Study the drawing (mm; zero at the part's minimum x, y, z) and answer. A direction names the side the tool comes from. Round coordinates to 2 decimals unless told otherwise and drop trailing zeros. Loops run counter-clockwise (first coordinate to the right, second up) from the corner with the lowest first, then second, coordinate; pieces in that order, holes last. Notation, with made-up numbers: M 46.25,42 L 71.25,42 A14 cw 71.25,59 Z; hole C -22.5,-15.75 d9. An arc over 180 degrees is marked long. Write each question's results on one line, items separated by ' | '.
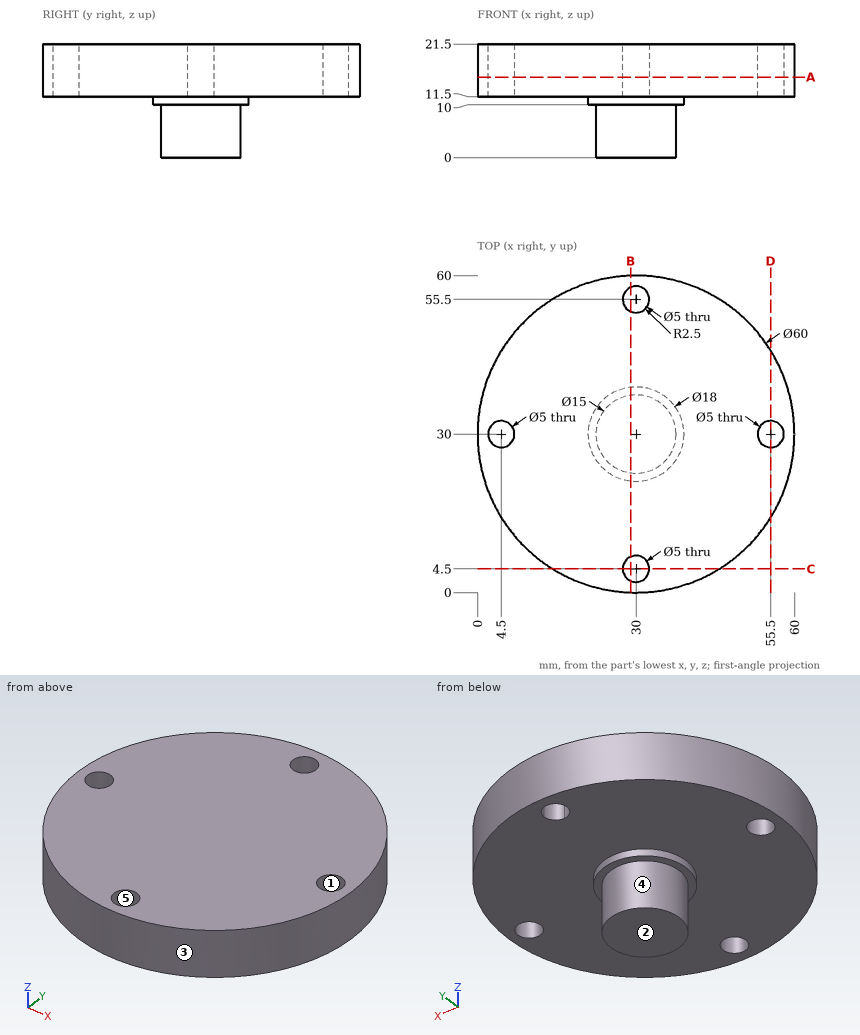
Item 1: For the marked faces 4 and 5, determine the directions among +Z, -Z, +X, -X, +Y, -Y from which every point of the face is accessible in a straight line to the end or side of a thin tool.
Outcome:
face 4: -Z | face 5: +Z, -Z
Item 2: The part is cut by section A-A (z = 15.25). Determine the outline of the cut face in (x, y).
Outcome:
outline: C 30,30 d60; hole C 4.5,30 d5; hole C 30,4.5 d5; hole C 30,55.5 d5; hole C 55.5,30 d5
Item 3: Straight lines are drawn through the part: line 1 (Y direction, x = 32, z = 12); line 2 (Z direction, x = 55, y = 27.5); line 3 (Y direction, x = 4.5, z = 16). For each, find the intervals that lie inside material, in ascending order.
Outcome:
line 1: y = 0.07 to 3, 6 to 54, 57 to 59.93 | line 2: z = 11.5 to 21.5 | line 3: y = 14.2 to 27.5, 32.5 to 45.8
Item 4: The part is cut by section C-C (y = 4.5). Determine the outline of the cut face in (x, z).
Outcome:
outline: M 14.2,11.5 L 27.5,11.5 L 27.5,21.5 L 14.2,21.5 Z; M 32.5,11.5 L 45.8,11.5 L 45.8,21.5 L 32.5,21.5 Z
Item 5: The mould has two halves that part along Y. Classify the marked faces 1, 2 and 3: pulls with the +Y half, pulls with the -Y half, needs draft (parallel to the pull), parting line crosses it, or undercut.
Outcome:
face 1: undercut | face 2: needs draft | face 3: parting line crosses it
Item 6: Flat-ended cylindrical pins translate along their axes: pin 1 (12 mm diameter, centred on x = 13, z = 9.5, fed in from +Y); pin 2 (6 mm diameter, centred on y = 38, z = 4, fed in from -X); pin 3 (12 mm diameter, centred on y = 37, z = 17.5, fed in from +X). Find the tip coordinate at first contact, or state that the pin passes through.
Outcome:
pin 1: stops at y = 57.77 | pin 2: stops at x = 24.41 | pin 3: stops at x = 59.98
Item 7: The part is cut by section B-B (x = 29). Determine the outline of the cut face in (y, z).
Outcome:
outline: M 0.02,11.5 L 2.21,11.5 L 2.21,21.5 L 0.02,21.5 Z; M 6.79,11.5 L 21.06,11.5 L 21.06,10 L 22.57,10 L 22.57,0 L 37.43,0 L 37.43,10 L 38.94,10 L 38.94,11.5 L 53.21,11.5 L 53.21,21.5 L 6.79,21.5 Z; M 57.79,11.5 L 59.98,11.5 L 59.98,21.5 L 57.79,21.5 Z
